The model under review builds one solid part; all positions refer to its coordinate system, in mm. A direction names the side the tool comes from. Coordinates: 2 decimals unless noted, no trailing zeros. Loops run counter-clockwise (first coordinate to the right, second up) from the corner with the lowest first, then second, coordinate; pieces in that order, holes last. Notation, with made-up numbers: M 56.25,-10.5 L 77.25,-10.5 A17 ccw 77.25,5.5 Z; hole C 62,56.25 d4. An arc over 180 degrees is marked long. Use one line per item in the form item = value.
```python
from build123d import *

# Parameters (mm, degrees)
SKETCH1_R           = 2.6035
BOSS_EXTRUDE1_DEPTH = 914.4
SKETCH2_W           = 591.784504761
SKETCH2_H           = 34.760821459
SKETCH2_W_2         = 1099.97900941
SKETCH2_H_2         = 36.169365112
CUT_EXTRUDE1_DEPTH  = 27.432


with BuildPart() as part:
    # Sketch1 → Boss-Extrude1 (new body, symmetric)
    with BuildSketch(Plane.XY):
        with BuildLine():
            Line((-7.179650497, -8.645192506), (-3.952270251, -5.423690499))
            ThreePointArc((-3.952270251, -5.423690499), (-2.922936451, -4.736929036), (-1.709253557, -4.4958))
            Line((-1.709253557, -4.4958), (1.709253557, -4.4958))
            ThreePointArc((1.709253557, -4.4958), (2.922936451, -4.736929036), (3.952270251, -5.423690499))
            Line((3.952270251, -5.423690499), (7.179650497, -8.645192506))
            ThreePointArc((7.179650497, -8.645192506), (7.41473083, -9.822813117), (6.416408329, -10.4902))
            Line((6.416408329, -10.4902), (4.287512407, -10.4902))
            ThreePointArc((4.287512407, -10.4902), (3.54574862, -10.79744862), (3.2385, -11.539212407))
            Line((3.2385, -11.539212407), (3.2385, -11.650987593))
            ThreePointArc((3.2385, -11.650987593), (3.54574862, -12.39275138), (4.287512407, -12.7))
            Line((4.287512407, -12.7), (5.317126718, -12.7))
            ThreePointArc((5.317126718, -12.7), (5.825126718, -12.192), (6.333126718, -12.7))
            Line((6.333126718, -12.7), (9.550443118, -12.7))
            ThreePointArc((9.550443118, -12.7), (10.058366869, -12.192000006), (10.566443095, -12.699847501))
            ThreePointArc((10.566443095, -12.699847501), (12.082537762, -12.08250727), (12.699846982, -10.566399977))
            ThreePointArc((12.699846982, -10.566399977), (12.192000006, -10.058323491), (12.7, -9.5504))
            Line((12.7, -9.5504), (12.7, -6.3330836))
            ThreePointArc((12.7, -6.3330836), (12.192, -5.8250836), (12.7, -5.3170836))
            Line((12.7, -5.3170836), (12.7, -4.287469289))
            ThreePointArc((12.7, -4.287469289), (12.39275138, -3.545705502), (11.650987593, -3.238456882))
            Line((11.650987593, -3.238456882), (11.539212407, -3.238456882))
            ThreePointArc((11.539212407, -3.238456882), (10.79744862, -3.545705502), (10.4902, -4.287469289))
            Line((10.4902, -4.287469289), (10.4902, -6.402089023))
            ThreePointArc((10.4902, -6.402089023), (9.856505071, -7.351067942), (8.737131347, -7.129408934))
            Line((8.737131347, -7.129408934), (5.441005833, -3.840816462))
            ThreePointArc((5.441005833, -3.840816462), (4.750877967, -2.809883091), (4.5085, -1.593185507))
            Line((4.5085, -1.593185507), (4.5085, 1.593185507))
            ThreePointArc((4.5085, 1.593185507), (4.750877967, 2.809883091), (5.441005833, 3.840816462))
            Line((5.441005833, 3.840816462), (8.737131347, 7.129408934))
            ThreePointArc((8.737131347, 7.129408934), (9.856505071, 7.351067942), (10.4902, 6.402089023))
            Line((10.4902, 6.402089023), (10.4902, 4.287469289))
            ThreePointArc((10.4902, 4.287469289), (10.79744862, 3.545705502), (11.539212407, 3.238456882))
            Line((11.539212407, 3.238456882), (11.650987593, 3.238456882))
            ThreePointArc((11.650987593, 3.238456882), (12.39275138, 3.545705502), (12.7, 4.287469289))
            Line((12.7, 4.287469289), (12.7, 5.3170836))
            ThreePointArc((12.7, 5.3170836), (12.192, 5.8250836), (12.7, 6.3330836))
            Line((12.7, 6.3330836), (12.7, 9.5504))
            ThreePointArc((12.7, 9.5504), (12.192000006, 10.058323491), (12.699846982, 10.566399977))
            ThreePointArc((12.699846982, 10.566399977), (12.082537762, 12.08250727), (10.566443095, 12.699847501))
            ThreePointArc((10.566443095, 12.699847501), (10.058366869, 12.192000006), (9.550443118, 12.7))
            Line((9.550443118, 12.7), (6.333126718, 12.7))
            ThreePointArc((6.333126718, 12.7), (5.825126718, 12.192), (5.317126718, 12.7))
            Line((5.317126718, 12.7), (4.287512407, 12.7))
            ThreePointArc((4.287512407, 12.7), (3.54574862, 12.39275138), (3.2385, 11.650987593))
            Line((3.2385, 11.650987593), (3.2385, 11.539212407))
            ThreePointArc((3.2385, 11.539212407), (3.54574862, 10.79744862), (4.287512407, 10.4902))
            Line((4.287512407, 10.4902), (6.476788598, 10.4902))
            ThreePointArc((6.476788598, 10.4902), (7.432222385, 9.85140422), (7.207036008, 8.724370562))
            Line((7.207036008, 8.724370562), (3.898272566, 5.423169045))
            ThreePointArc((3.898272566, 5.423169045), (2.869120213, 4.736787962), (1.655778399, 4.4958))
            Line((1.655778399, 4.4958), (-1.655778399, 4.4958))
            ThreePointArc((-1.655778399, 4.4958), (-2.869120213, 4.736787962), (-3.898272566, 5.423169045))
            Line((-3.898272566, 5.423169045), (-7.207036008, 8.724370562))
            ThreePointArc((-7.207036008, 8.724370562), (-7.432222385, 9.85140422), (-6.476788598, 10.4902))
            Line((-6.476788598, 10.4902), (-4.287512407, 10.4902))
            ThreePointArc((-4.287512407, 10.4902), (-3.54574862, 10.79744862), (-3.2385, 11.539212407))
            Line((-3.2385, 11.539212407), (-3.2385, 11.650987593))
            ThreePointArc((-3.2385, 11.650987593), (-3.54574862, 12.39275138), (-4.287512407, 12.7))
            Line((-4.287512407, 12.7), (-5.317126718, 12.7))
            ThreePointArc((-5.317126718, 12.7), (-5.825126718, 12.192), (-6.333126718, 12.7))
            Line((-6.333126718, 12.7), (-9.550443118, 12.7))
            ThreePointArc((-9.550443118, 12.7), (-10.058366869, 12.192000006), (-10.566443095, 12.699847501))
            ThreePointArc((-10.566443095, 12.699847501), (-12.082537762, 12.08250727), (-12.699846982, 10.566399977))
            ThreePointArc((-12.699846982, 10.566399977), (-12.192000006, 10.058323491), (-12.7, 9.5504))
            Line((-12.7, 9.5504), (-12.7, 6.3330836))
            ThreePointArc((-12.7, 6.3330836), (-12.192, 5.8250836), (-12.7, 5.3170836))
            Line((-12.7, 5.3170836), (-12.7, 4.287469289))
            ThreePointArc((-12.7, 4.287469289), (-12.39275138, 3.545705502), (-11.650987593, 3.238456882))
            Line((-11.650987593, 3.238456882), (-11.539212407, 3.238456882))
            ThreePointArc((-11.539212407, 3.238456882), (-10.79744862, 3.545705502), (-10.4902, 4.287469289))
            Line((-10.4902, 4.287469289), (-10.4902, 6.402089023))
            ThreePointArc((-10.4902, 6.402089023), (-9.856505071, 7.351067942), (-8.737131347, 7.129408934))
            Line((-8.737131347, 7.129408934), (-5.441005833, 3.840816462))
            ThreePointArc((-5.441005833, 3.840816462), (-4.750877967, 2.809883091), (-4.5085, 1.593185507))
            Line((-4.5085, 1.593185507), (-4.5085, -1.593185507))
            ThreePointArc((-4.5085, -1.593185507), (-4.750877967, -2.809883091), (-5.441005833, -3.840816462))
            Line((-5.441005833, -3.840816462), (-8.737131347, -7.129408934))
            ThreePointArc((-8.737131347, -7.129408934), (-9.856505071, -7.351067942), (-10.4902, -6.402089023))
            Line((-10.4902, -6.402089023), (-10.4902, -4.287469289))
            ThreePointArc((-10.4902, -4.287469289), (-10.79744862, -3.545705502), (-11.539212407, -3.238456882))
            Line((-11.539212407, -3.238456882), (-11.650987593, -3.238456882))
            ThreePointArc((-11.650987593, -3.238456882), (-12.39275138, -3.545705502), (-12.7, -4.287469289))
            Line((-12.7, -4.287469289), (-12.7, -5.3170836))
            ThreePointArc((-12.7, -5.3170836), (-12.192, -5.8250836), (-12.7, -6.3330836))
            Line((-12.7, -6.3330836), (-12.7, -9.5504))
            ThreePointArc((-12.7, -9.5504), (-12.192000006, -10.058323491), (-12.699846982, -10.566399977))
            ThreePointArc((-12.699846982, -10.566399977), (-12.082537762, -12.08250727), (-10.566443095, -12.699847501))
            ThreePointArc((-10.566443095, -12.699847501), (-10.058366869, -12.192000006), (-9.550443118, -12.7))
            Line((-9.550443118, -12.7), (-6.333126718, -12.7))
            ThreePointArc((-6.333126718, -12.7), (-5.825126718, -12.192), (-5.317126718, -12.7))
            Line((-5.317126718, -12.7), (-4.287512407, -12.7))
            ThreePointArc((-4.287512407, -12.7), (-3.54574862, -12.39275138), (-3.2385, -11.650987593))
            Line((-3.2385, -11.650987593), (-3.2385, -11.539212407))
            ThreePointArc((-3.2385, -11.539212407), (-3.54574862, -10.79744862), (-4.287512407, -10.4902))
            Line((-4.287512407, -10.4902), (-6.416408329, -10.4902))
            ThreePointArc((-6.416408329, -10.4902), (-7.41473083, -9.822813117), (-7.179650497, -8.645192506))
        make_face()
        Circle(SKETCH1_R, mode=Mode.SUBTRACT)
    extrude(amount=BOSS_EXTRUDE1_DEPTH, both=True)

    # Sketch2 → Cut-Extrude1 (cut)
    with BuildSketch(Plane(origin=(12.7, 0, 0), x_dir=(0, 0, -1), z_dir=(1, 0, 0))):
        with Locations((-622.565020226, -0.58573738)):
            Rectangle(SKETCH2_W, SKETCH2_H)
        with Locations((375.067711741, 0.118534447)):
            Rectangle(SKETCH2_W_2, SKETCH2_H_2)
    extrude(amount=-CUT_EXTRUDE1_DEPTH, mode=Mode.SUBTRACT)


solid = part.part
```
1. Add section A-A (x = 0). State the section outline as (y, z) points.
Response values:
outline = M -4.5,174.92 L -2.6,174.92 L -2.6,326.67 L -4.5,326.67 Z; M 2.6,174.92 L 4.5,174.92 L 4.5,326.67 L 2.6,326.67 Z
2. Add section B-B (y = 0). State the section outline as (x, z) points, then the cut area to 3 significant figures.
Response values:
outline = M -4.51,174.92 L -2.6,174.92 L -2.6,326.67 L -4.51,326.67 Z; M 2.6,174.92 L 4.51,174.92 L 4.51,326.67 L 2.6,326.67 Z
area = 578 mm^2
3. Wall thickness on line 1 along Y through (x, z) = (0, 263.5); line 2 along X through (y, z) = (9, 192); line 3 along X through (y, z) = (0, 252.5): over which ranges is each line inside the solid? List them lowest first. Write a range as from..to.
Response values:
line_1 = -4.5..-2.6, 2.6..4.5
line_2 = -12.7..-7.4, 7.4..12.7
line_3 = -4.51..-2.6, 2.6..4.51
4. Machinability: for faces 1 (the face through (-4.508, 0, 252)), 2 (the face through (0, -4.496, 252)), 3 (the face through (7.112, -5.508, 251.86)), which of the approach directions +Z, -Z, +X, -X, +Y, -Y give a long, thin tool a straight path to every point of the face, cutting with its end or side? Answer none if there is none.
Response values:
face_1 = +Z, -Z, -X
face_2 = +Z, -Z, -Y
face_3 = +Z, -Z
5. The part is to be moulded in two halves that separate along X. For faces 4 (the face through (12.7, -8, 252)), 5 (the face through (-12.7, 8, 252)), 6 (the face through (-7.066, -5.462, 251.86)), say which applies: pulls with the +X half, pulls with the -X half, needs draft (parallel to the pull), parting line crosses it, or undercut.
Response values:
face_4 = pulls with the +X half
face_5 = pulls with the -X half
face_6 = undercut
6. Insertion check: P1, Ø1.6, axis at y = -0.5, z = 234.5, coming from the -X side; P2, Ø1, axis at y = 1, z = 234.5, coming from the +X side; P3, Ø2.5, axis at x = 0, z = 243, coming from the -Y side. Each pin has a flat end and moves straight along its axis. Give the tip position at first contact, or say it passes through.
Response values:
P1 = -4.51
P2 = 4.51
P3 = -4.5
